Verification items for the finished model (mm, model axes). Give positions to 0.01 mm unless a question says otherwise; leave off trailing zeros. Write each loop counter-clockwise with the first axis right and the second up, starting at its lowest first coordinate (ties: lowest second). Pieces come first, ordered by that corner, then holes. Notation, with made-up numbers: M -2,65 L 13,65 A18 ccw 13,100 Z; hole C 88.5,11 d5. An arc over 180 degrees is marked long. Write item = value, one per line.
from build123d import *

# Parameters (mm, degrees)
ESQUISSE1_W             = 17
ESQUISSE1_H             = 181
BOSS_EXTRU_1_DEPTH      = 10
ESQUISSE2_R             = 1.5
ENL_V_MAT_EXTRU_1_DEPTH = 5
ESQUISSE4_R             = 1.5
ENL_V_MAT_EXTRU_2_DEPTH = 5


with BuildPart() as part:
    # Esquisse1 → Boss.-Extru.1 (new body)
    with BuildSketch(Plane.XY):
        Rectangle(ESQUISSE1_W, ESQUISSE1_H)
    extrude(amount=BOSS_EXTRU_1_DEPTH)

    # Esquisse2 → Enlèv. mat.-Extru.1 (cut)
    with BuildSketch(Plane.XY.offset(10)):
        with Locations((0, 47.5)):
            Circle(ESQUISSE2_R)
        with Locations((0, -80.5)):
            Circle(ESQUISSE2_R)
    extrude(amount=-ENL_V_MAT_EXTRU_1_DEPTH, mode=Mode.SUBTRACT)

    # Esquisse4 → Enlèv. mat.-Extru.2 (cut)
    with BuildSketch(Plane(origin=(0, 0, 0), x_dir=(-1, 0, 0), z_dir=(0, 0, -1))):
        with Locations((0, 14.5)):
            Circle(ESQUISSE4_R)
        with Locations((0, -40.5)):
            Circle(ESQUISSE4_R)
    extrude(amount=-ENL_V_MAT_EXTRU_2_DEPTH, mode=Mode.SUBTRACT)


solid = part.part
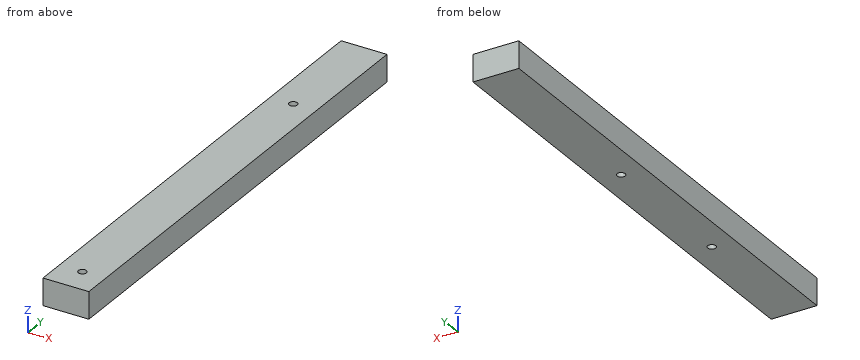
1) Material ranges on probe 1 along Y at (x, z) = (0, 6.9); probe 2 along Y at (x, z) = (0, 2.55); probe 3 along X at (y, z) = (-80.5, 6.9), recorded low to high. Write a range as from..to.
From the geometry:
probe_1 = -90.5..-82, -79..46, 49..90.5
probe_2 = -90.5..-42, -39..13, 16..90.5
probe_3 = -8.5..-1.5, 1.5..8.5
2) Cross-section at A-A on x = 0. Record the boundary of the cut face in (y, z).
From the geometry:
outline = M -90.5,0 L -42,0 L -42,5 L -39,5 L -39,0 L 13,0 L 13,5 L 16,5 L 16,0 L 90.5,0 L 90.5,10 L 49,10 L 49,5 L 46,5 L 46,10 L -79,10 L -79,5 L -82,5 L -82,10 L -90.5,10 Z
3) Cross-section at B-B on y = 47.5. Record the boundary of the cut face in (x, z).
From the geometry:
outline = M -8.5,0 L 8.5,0 L 8.5,10 L 1.5,10 L 1.5,5 L -1.5,5 L -1.5,10 L -8.5,10 Z
4) Depth check by flat-ended pin: P1, Ø2.5, axis at x = 0, y = 14.5, coming from the -Z side. Enter the tip coordinate at first touch or a pass-through.
From the geometry:
P1 = 5
